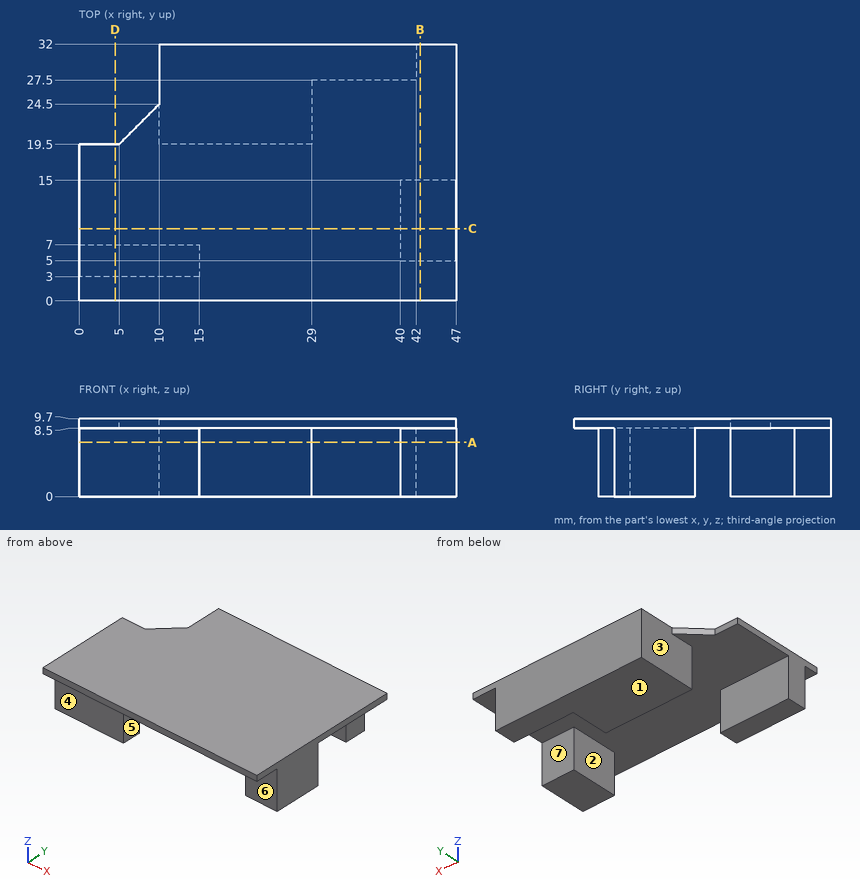
Can you work these out from the drawing? Everything is in mm from the part's minimum corner. A direction names the side the tool comes from. Coordinates: 2 decimals unless noted, no trailing zeros. Loops run counter-clockwise (first coordinate to the right, second up) from the corner with the lowest first, then second, coordinate; pieces in that order, holes last.
1) I need wall thicknesses on probe 1 along Y at (x, z) = (40.5, 4.5); probe 2 along X at (y, z) = (5.5, 1.25); probe 3 along Y at (x, z) = (39.5, 5.5). Which ranges of each line are inside material? Lowest first, please.
2) Thinking about a two-plate mould opening in X: for the marked faces 1, 2 and 3, which applies, pulls with the +X half, pulls with the -X half, needs draft (parallel to the pull), parting line crosses it, or undercut?
3) Which directions (+Z, -Z, +X, -X, +Y, -Y) give clear straight access to the entire face, cutting with the end or side of a thin tool? Please do the marked faces 4, 5, 6 and 7.
4) For pin 1 (4 mm diameter, centred on y = 24, z = 3, fed in from +X); pin 2 (1.5 mm diameter, centred on x = 36, y = 14, fed in from -Z); pin 3 (4 mm diameter, centred on x = 16.5, z = 4.5, fed in from -Y), each with a flat end and sliding along its axis, tell me the tip position at first contact or that it passes through.
5) Imagine slicing it at D-D on x = 4.5. List the corners of the cut face in (y, z) for me, plus the area to 3 significant figures.
6) Imagine slicing it at B-B on x = 42.5. List the corners of the cut face in (y, z) for me, plus the area to 3 significant figures.
7) Imagine slicing it at C-C on y = 9. List the corners of the cut face in (x, z) for me.
8) Imagine slicing it at A-A on z = 6.75. List the corners of the cut face in (x, y) for me, plus the area to 3 significant figures.
Completed:
1. probe 1: y = 5 to 15, 27.5 to 32
1. probe 2: x = 0 to 15, 40 to 47
1. probe 3: y = 27.5 to 32
2. face 1: needs draft
2. face 2: undercut
2. face 3: pulls with the -X half
3. face 4: -Z, +X, -X, -Y
3. face 5: -Z, -Y
3. face 6: -Z, +X, -Y
3. face 7: -Z, +X, -X
4. pin 1: stops at x = 29
4. pin 2: stops at z = 8.5
4. pin 3: stops at y = 3
5. outline: (0, 8.5) - (3, 8.5) - (3, 0) - (7, 0) - (7, 8.5) - (19.5, 8.5) - (19.5, 9.7) - (0, 9.7) - close
5. area: 57.4 mm2
6. outline: (0, 8.5) - (5, 8.5) - (5, 0) - (15, 0) - (15, 8.5) - (32, 8.5) - (32, 9.7) - (0, 9.7) - close
6. area: 123 mm2
7. outline: (0, 8.5) - (40, 8.5) - (40, 0) - (47, 0) - (47, 9.7) - (0, 9.7) - close
8. outline: (0, 3) - (15, 3) - (15, 7) - (0, 7) - close; (10, 19.5) - (29, 19.5) - (29, 27.5) - (42, 27.5) - (42, 32) - (10, 32) - close; (40, 5) - (47, 5) - (47, 15) - (40, 15) - close
8. area: 426 mm2
